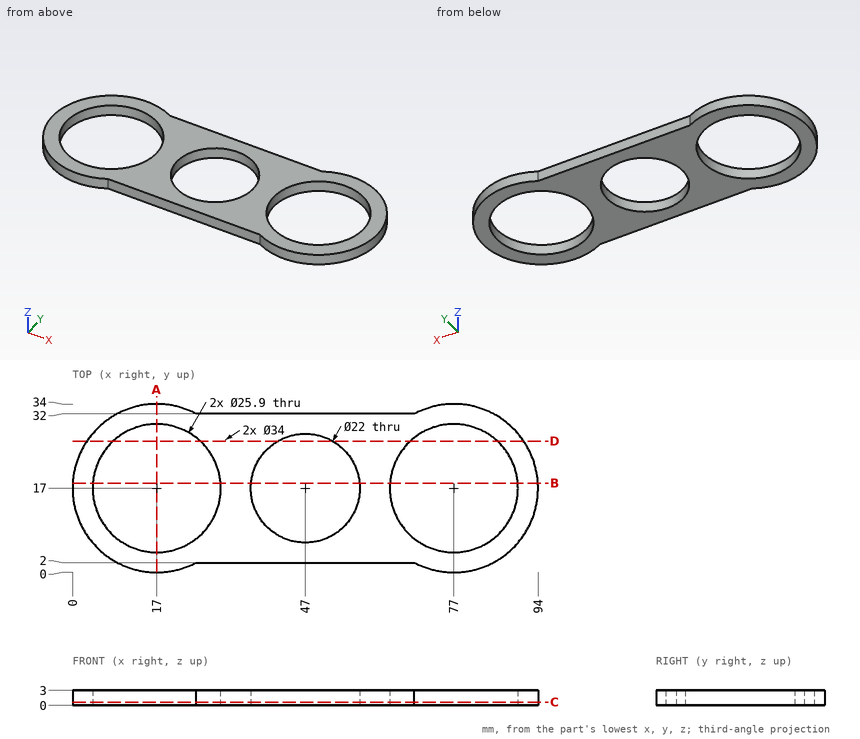
Check sheet for the drawn part. Datum: minimum x, y, z corner. Units: mm. Round coordinates to 2 decimals unless told otherwise and drop trailing zeros. Order: outer loops, then holes, each group sorted by start corner. A loop starts at its lowest first (then second) coordinate and runs counter-clockwise, first axis right, second up. Notation, with made-up numbers: (20, -38) -> (68, -38) arc R21 ccw to (68, -9) -> close; hole circle Ø10 at (-19.5, -5). An arc over 180 degrees is marked (long way). Put each result on its own line as item: value.
1) Section check D-D (y = 26.5). Record the cut outline in (x, z).
Final values:
outline: (2.9, 0) -> (8.2, 0) -> (8.2, 3) -> (2.9, 3) -> close; (25.8, 0) -> (41.45, 0) -> (41.45, 3) -> (25.8, 3) -> close; (52.55, 0) -> (68.2, 0) -> (68.2, 3) -> (52.55, 3) -> close; (85.8, 0) -> (91.1, 0) -> (91.1, 3) -> (85.8, 3) -> close
2) Depth check by flat-ended pin: pin 1 (1.5 mm diameter, centred on y = 12.5, z = 2.5, fed in from +X); pin 2 (1 mm diameter, centred on y = 23, z = 1.5, fed in from +X); pin 3 (1.5 mm diameter, centred on x = 48.5, z = 2, fed in from +Y). Enter the tip coordinate at first touch or a pass-through.
Final values:
pin 1: stops at x = 93.58
pin 2: stops at x = 93.09
pin 3: stops at y = 32
3) Material ranges on line 1 (Y direction, x = 17, z = 1.35); line 2 (X direction, y = 10.5, z = 0.3); line 3 (X direction, y = 8.5, z = 1.4), recorded low to high.
Final values:
line 1: y = 0 to 4.05, 29.95 to 34
line 2: x = 1.29 to 5.8, 28.2 to 38.13, 55.87 to 65.8, 88.2 to 92.71
line 3: x = 2.28 to 7.23, 26.77 to 40.02, 53.98 to 67.23, 86.77 to 91.72
4) Section check C-C (z = 0.65). Record the cut outline in (x, y).
Final values:
outline: (25, 2) -> (69, 2) arc R17 ccw (long way) to (69, 32) -> (25, 32) arc R17 ccw (long way) to start; hole circle Ø25.9 at (17, 17); hole circle Ø22 at (47, 17); hole circle Ø25.9 at (77, 17)
5) Section check A-A (x = 17). Record the cut outline in (y, z).
Final values:
outline: (0, 0) -> (4.05, 0) -> (4.05, 3) -> (0, 3) -> close; (29.95, 0) -> (34, 0) -> (34, 3) -> (29.95, 3) -> close
6) Section check B-B (y = 18). Record the cut outline in (x, z).
Final values:
outline: (0.03, 0) -> (4.09, 0) -> (4.09, 3) -> (0.03, 3) -> close; (29.91, 0) -> (36.05, 0) -> (36.05, 3) -> (29.91, 3) -> close; (57.95, 0) -> (64.09, 0) -> (64.09, 3) -> (57.95, 3) -> close; (89.91, 0) -> (93.97, 0) -> (93.97, 3) -> (89.91, 3) -> close
